Can you work these out from the model? Positions are in its coordinate system, mm. A direction names the side the tool comes from. Give positions to 0.01 mm unless a question says otherwise; leave off trailing zeros. Write each loop counter-clockwise with the first axis right and the second up, starting at its lowest first coordinate (ties: lowest second). Pieces come first, ordered by that corner, then holes. Notation, with made-up numbers: (-27.5, -2.5) -> (-9.5, -2.5) arc R19 cw to (-9.5, 2.5) -> close; hole circle Ø10 at (74.25, 29). An arc over 180 degrees is marked (long way). Answer as CSV lines item,"result". Start each with the question number.
1. If we section it at D-D on x = 79: Write out the boundary of the cut face in (y, z).
2. If we section it at C-C on z = -41: Write out the boundary of the cut face in (x, y), plus the area to 3 significant figures.
3. I need wall thicknesses on line 1 (Y direction, x = 10, z = 122.8); line 2 (Z direction, x = 105, y = 130.5); line 3 (X direction, y = 65, z = 53.5). Which ranges of each line are inside material? Lowest first, please. Write a range as [from, to].
4. On a 3-axis mill with a long thin cutter (end or side, diameter ignored), from which of +Z, -Z, +X, -X, +Y, -Y can I reach the whole of each face in a straight line? I mean faces 1 (the face through (90.97, 131.24, 70.29)), 2 (the face through (114.022, 94.3, 32.753)). Say none if no direction works.
5. If we section it at B-B on y = 76: Write out the boundary of the cut face in (x, z).
6. If we mould it in two halves opening along Z, with no side actions, what happens to faces 3 (the face through (110.723, 104.14, -53.937)), 4 (the face through (109.158, 94.3, 60.906)), 5 (the face through (99, 45, 52)), 6 (the face through (85.357, 94.3, 82.166))? For each: pulls with the +Z half, pulls with the -Z half, needs draft (parallel to the pull), parting line crosses it, or undercut.
7. I'm going to push flat-ended pins straight in: P1, Ø1.5, axis at y = 119, z = 100, coming from the -X side; P2, Ø5, axis at x = 74, y = 59, coming from the -Z side; P3, Ø3, axis at x = 53, y = 56, coming from the -Z side; P4, Ø2.5, axis at x = 10, y = 105, coming from the -Z side. Where does each tip first touch, or does it pass through?
8. If we section it at A-A on y = 53: Write out the boundary of the cut face in (x, z).
Autodesk Inventor part; units mm, degrees
ref_plane "YZ Plane" through (0, 0, 0) normal (1, 0, 0) x (0, 1, 0)
ref_plane "XZ Plane" through (0, 0, 0) normal (0, 1, 0) x (-1, 0, 0)
ref_plane "XY Plane" through (0, 0, 0) normal (0, 0, 1) x (1, 0, 0)
sketch "スケッチ1" plane through (0, 0, 0) normal (0, 1, 0) x (-1, 0, 0)
  circle A0 centre (0, 0) radius 125
  dimension "d0" = 250
extrude "押し出し1" add sketch "スケッチ1" along normal blind 375
sketch "スケッチ2" plane through (0, 0, 0) normal (0, -1, 0) x (1, 0, 0)
  circle A0 centre (0, 0) radius 125
extrude "押し出し2" cut sketch "スケッチ2" against normal blind 40
sketch "スケッチ3" plane through (0, 40, 0) normal (0, -1, 0) x (1, 0, 0)
  circle A0 centre (0, 0) radius 125
  point P0 (0, 100)
  point P1 (-86.6025, -50)
  point P2 (86.6025, -50)
  dimension "d5" = 100
  dimension "d8" = 360
hole "穴1" at (0, 40, 100) at (-86.6025, 40, -50) at (86.6025, 40, -50) direction (0, 1, 0) diameter 3.2 depth 8
sketch "スケッチ4" plane through (0, 40, 0) normal (0, -1, 0) x (1, 0, 0)
  circle A0 centre (0, 100) radius 1.6
  point P0 (0, 0)
  point P1 (0, 110)
  point P2 (-95.2628, -55)
  point P3 (95.2628, -55)
  dimension "d17" = 10
  dimension "d20" = 360
hole "穴2" at (0, 40, 110) at (-95.2628, 40, -55) at (95.2628, 40, -55) direction (0, 1, 0) diameter 3.2 depth 8
sketch "スケッチ5" plane through (0, 375, 0) normal (0, 1, 0) x (1, 0, 0)
  circle A0 centre (0, 0) radius 120
  dimension "d29" = 240
extrude "押し出し3" cut sketch "スケッチ5" against normal blind 330
sketch "スケッチ6" plane through (0, 45, 0) normal (0, 1, 0) x (1, 0, 0)
  circle A0 centre (0, 0) radius 120
  line L0 (0, -118) -> (-21.8174, -118)
  line L1 (0, -118) -> (21.8174, -118)
  arc A1 (21.8174, -118) -> (-21.8174, -118) centre (0, 0) ccw
  arc A2 (-21.8174, -118) -> (21.8174, -118) centre (0, 0) ccw
  arc A3 (113.0997, 40.1056) -> (91.2823, 77.8944) centre (0, 0) ccw
  line L2 (102.191, 59) -> (91.2823, 77.8944)
  line L3 (102.191, 59) -> (113.0997, 40.1056)
  arc A4 (-91.2823, 77.8944) -> (-113.0997, 40.1056) centre (0, 0) ccw
  line L4 (-102.191, 59) -> (-113.0997, 40.1056)
  line L5 (-102.191, 59) -> (-91.2823, 77.8944)
  point P0 (-91.2823, 77.8944)
  point P1 (-113.0997, 40.1056)
  point P2 (113.0997, 40.1056)
  point P3 (91.2823, 77.8944)
  dimension "d32" = 118
  dimension "d35" = 360
extrude "押し出し4" add sketch "スケッチ6" along normal blind 330 contours L3 L2 A0 | A0 L0 L1 | L5 L4 A0
sketch "スケッチ8" plane through (21.8174, 45, 118) normal (0, 0, -1) x (-1, 0, 0)
  line L0 (43.6348, 0) -> (0, 0)
  point P0 (21.8174, -45)
  point P1 (11.8174, 60)
  point P2 (31.8174, 60)
  point P3 (11.8174, 90)
  point P4 (31.8174, 90)
  dimension "d52" = 30
  dimension "d90" = 60
  dimension "d91" = 60
  dimension "d92" = 30
hole "穴4" at (10, 105, 118) at (-10, 105, 118) at (10, 135, 118) at (-10, 135, 118) direction (0, 0, 1) diameter 3.2 depth 8
sketch "スケッチ11" plane through (113.0997, 45, -40.1056) normal (-0.8660254, 0, 0.5) x (0.5, 0, 0.8660254)
  line L0 (0, 0) -> (-43.6348, 0)
  point P0 (-21.8174, -45)
  point P1 (-31.8174, 60)
  point P2 (-31.8174, 90)
  point P3 (-11.8174, 60)
  point P4 (-11.8174, 90)
  dimension "d65" = 30
  dimension "d95" = 60
  dimension "d96" = 60
  dimension "d98" = 30
hole "穴5" at (97.191, 105, -67.6603) at (97.191, 135, -67.6603) at (107.191, 135, -50.3397) at (107.191, 105, -50.3397) direction (0.8660254, 0, -0.5) diameter 3.2 depth 8
sketch "スケッチ12" plane through (0, 375, 0) normal (0, 1, 0) x (1, 0, 0)
  circle A0 centre (0, 0) radius 121.5
  dimension "d73" = 243
extrude "押し出し6" cut sketch "スケッチ12" against normal blind 330
sketch "スケッチ13" plane through (0, 375, 0) normal (0, 1, 0) x (1, 0, 0)
  circle A0 centre (0, 0) radius 125
  line L0 (0, -125) -> (0, 0)
  line L1 (0, 0) -> (108.2532, 62.5)
  arc A1 (0, -125) -> (108.2532, 62.5) centre (0, 0) ccw
  circle A2 centre (0, 0) radius 125
  dimension "d76" = 125
  dimension "d77" = 120
extrude "押し出し7" cut sketch "スケッチ13" against normal blind 400 contours L1 L0 A0 picked at (69.3351, 45.9431)
sketch "スケッチ14" plane through (0, 45, 0) normal (0, 1, 0) x (1, 0, 0)
  line L0 (0, 0) -> (85.2169, 49.2)
  line L1 (0, -111.6) -> (0, -121.5)
  circle A0 centre (0, 0) radius 121.5
extrude "押し出し8" cut sketch "スケッチ14" against normal blind 400
sketch "スケッチ15" plane through (0, 40, 0) normal (0, -1, 0) x (1, 0, 0)
  line L0 (0, 0) -> (105.2221, 60.75)
  arc A0 (105.2221, -60.75) -> (0, 121.5) centre (0, 0) ccw
  line L1 (0, 0) -> (121.5, 0) construction
  line L2 (102.9357, 59.43) -> (115.531, 37.6143)
  line L3 (102.9357, 59.43) -> (90.3404, 81.2456)
  dimension "d82" = 30
extrude "押し出し9" add sketch "スケッチ15" against normal blind 335
sketch "スケッチ17" plane through (0, 40, 0) normal (0, -1, 0) x (1, 0, 0)
  circle A0 centre (0, 0) radius 125
extrude "押し出し11" cut sketch "スケッチ17" against normal blind 5
sketch "スケッチ19" plane through (0, 375, 0) normal (0, 1, 0) x (1, 0, 0)
  arc A0 (115.531, -37.6143) -> (105.2221, 60.75) centre (0, 0) ccw
  line L0 (115.531, -37.6143) -> (90.3404, -81.2456)
  line L1 (115.531, -37.6143) -> (90.3404, -81.2456)
  line L2 (90.3404, -81.2456) -> (81.6802, -76.2456)
  line L3 (115.531, -37.6143) -> (106.8708, -32.6143)
  line L4 (106.8708, -32.6143) -> (81.6802, -76.2456)
  dimension "d104" = 10
extrude "押し出し13" add sketch "スケッチ19" against normal blind 330
sketch "スケッチ21" plane through (0, 375, 0) normal (0, 1, 0) x (1, 0, 0)
  circle A0 centre (0, 0) radius 125
extrude "押し出し15" cut sketch "スケッチ21" against normal blind 230
fillet "フィレット1" radius 8 2 edges at (115.531, 95, 37.6143) (90.3404, 95, 81.2456)
sketch "スケッチ22" plane through (106.8708, 45, 32.6143) normal (-0.8660254, 0, -0.5) x (-0.5, 0, 0.8660254)
  line L0 (50.3812, 100) -> (0, 100)
  line L1 (25.1906, 85) -> (25.1906, 80.9836)
  point P0 (25.1906, -45)
  point P1 (10.1906, 85)
  point P2 (10.1906, 70)
  point P3 (40.1906, 85)
  point P4 (40.1906, 70)
  dimension "d112" = 15
  dimension "d113" = 15
  dimension "d114" = 15
hole "穴6" at (94.2755, 130, 54.43) at (101.7755, 130, 41.4396) at (101.7755, 115, 41.4396) at (86.7755, 130, 67.4204) at (86.7755, 115, 67.4204) direction (0.8660254, 0, 0.5) diameter 2.6 depth 10
sketch "スケッチ23" plane through (0, 45, 0) normal (0, -1, 0) x (1, 0, 0)
  line L0 (81.6802, 76.2456) -> (106.8708, 32.6143)
  arc A0 (118.386, 27.3315) -> (106.8708, 32.6143) centre (110.591, 25.5319) ccw
  line L1 (106.8708, 32.6143) -> (94.2755, 54.4299)
  line L2 (102.2857, 60.5558) -> (93.6255, 55.5558)
  line L3 (94.2755, 54.43) -> (101.2037, 58.43)
  line L4 (103.5857, 58.3041) -> (94.9255, 53.3041)
  line L5 (94.2755, 54.43) -> (102.2755, 54.43) construction
  point P0 (0, 0)
  dimension "d124" = 25.1905
  dimension "d126" = 8
  dimension "d127" = 30
hole "穴7" at (101.2037, 45, 58.43) direction (0, 1, 0) diameter 2.6 depth 10
sketch "スケッチ24" plane through (0, 45, 0) normal (0, -1, 0) x (1, 0, 0)
  circle A0 centre (101.2037, 58.43) radius 1.3
  line L0 (101.2037, 58.43) -> (96.2037, 67.0902)
  line L1 (94.7857, 73.5462) -> (86.1255, 68.5462)
  line L2 (101.2037, 58.43) -> (111.2037, 58.43) construction
  line L3 (96.2037, 67.0902) -> (106.2037, 49.7697)
  point P0 (0, 0)
  dimension "d135" = 10
  dimension "d136" = 120
  dimension "d137" = 20
hole "穴8" at (96.2037, 45, 67.0902) at (106.2037, 45, 49.7697) direction (0, 1, 0) diameter 2.6 depth 10
properties part number "newbody5"
Computed values:
1,outline,"(45, 92.31) -> (145, 92.31) -> (145, 96.87) -> (45, 96.87) -> close"
2,outline,"(114.37, 45) -> (118.08, 45) -> (118.08, 145) -> (114.37, 145) -> close"
2,area,"371 mm2"
3,line 1,"y = [45, 103.4], [106.6, 133.4], [136.6, 145]"
3,line 2,"z = [35.85, 41.92], [44.69, 67.82]"
3,line 3,"x = [94.81, 112.97]"
4,face 1,"none"
4,face 2,"+Y, -Y"
5,outline,"(0, 121.5) arc R121.5 cw to (82.86, 88.86) arc R8 cw to (81.68, 76.25) -> (106.87, 32.61) arc R8 cw to (118.39, 27.32) arc R121.5 cw to (105.22, -60.75) -> (108.25, -62.5) arc R125 ccw to (0, 125) -> close"
6,face 3,"undercut"
6,face 4,"parting line crosses it"
6,face 5,"needs draft"
6,face 6,"undercut"
7,P1,"stops at x = 67.91"
7,P2,"stops at z = 94.39"
7,P3,"stops at z = 108.59"
7,P4,"passes through"
8,outline,"(0, 121.5) arc R121.5 cw to (82.86, 88.86) arc R8 cw to (81.68, 76.25) -> (106.87, 32.61) arc R8 cw to (118.39, 27.32) arc R121.5 cw to (105.22, -60.75) -> (108.25, -62.5) arc R125 ccw to (0, 125) -> close; hole circle Ø2.6 at (96.2, 67.09); hole circle Ø2.6 at (101.2, 58.43); hole circle Ø2.6 at (106.2, 49.77)"
